from build123d import *

# Parameters (mm, degrees)
SKETCH1_R                 = 36
BIG_END_DEPTH             = 11
SKETCH2_R                 = 18
SMALL_END_DEPTH           = 11
BEAM_DEPTH                = 11
CAP_BOLT_BOSSES_DEPTH     = 11
BEAM_START                = 7
BEAM_POCKET_FRONT_DEPTH   = 5
BEAM_START_2              = -12
BEAM_POCKET_REAR_DEPTH    = 5
BIG_END_BORE_DEPTH        = 178.709988464
BIG_END_BORE_DEPTH_BACK   = 178.709988464
SKETCH7_R                 = 26.75
SMALL_END_BORE_DEPTH      = 178.709988464
SMALL_END_BORE_DEPTH_BACK = 178.709988464
SKETCH8_R                 = 11.85


with BuildPart() as part:
    # Sketch1 → Big End (new, symmetric)
    with BuildSketch(Plane.XY):
        Circle(SKETCH1_R)
    extrude(amount=BIG_END_DEPTH, both=True)



with BuildPart() as body_2:
    # Sketch2 → Small End (new, symmetric)
    with BuildSketch(Plane.XY):
        with Locations((0, 154.8)):
            Circle(SKETCH2_R)
    extrude(amount=SMALL_END_DEPTH, both=True)


with BuildPart() as part_1:
    add(part.part)

    add(body_2.part)  # Beam merges body 2
    # Sketch3 → Beam (add, symmetric)
    with BuildSketch(Plane.XY):
        Polygon((-15, 20), (15, 20), (10, 142.8), (-10, 142.8), align=None)
    extrude(amount=BEAM_DEPTH, both=True)

    # Sketch4 → Cap Bolt Bosses (add, symmetric)
    with BuildSketch(Plane.XY):
        with BuildLine():
            Line((29, -9), (37, -9))
            ThreePointArc((37, -9), (39.121320344, -8.121320344), (40, -6))
            Line((40, -6), (40, 9))
            ThreePointArc((40, 9), (39.121320344, 11.121320344), (37, 12))
            Line((37, 12), (29, 12))
            ThreePointArc((29, 12), (26.878679656, 11.121320344), (26, 9))
            Line((26, 9), (26, -6))
            ThreePointArc((26, -6), (26.878679656, -8.121320344), (29, -9))
        make_face()
        with BuildLine():
            Line((-37, -9), (-29, -9))
            ThreePointArc((-29, -9), (-26.878679656, -8.121320344), (-26, -6))
            Line((-26, -6), (-26, 9))
            ThreePointArc((-26, 9), (-26.878679656, 11.121320344), (-29, 12))
            Line((-29, 12), (-37, 12))
            ThreePointArc((-37, 12), (-39.121320344, 11.121320344), (-40, 9))
            Line((-40, 9), (-40, -6))
            ThreePointArc((-40, -6), (-39.121320344, -8.121320344), (-37, -9))
        make_face()
    extrude(amount=CAP_BOLT_BOSSES_DEPTH, both=True)

    # Sketch5 → Beam Pocket Front (cut)
    with BuildSketch(Plane.XY.offset(BEAM_START)):
        with BuildLine():
            Line((-5.386546762, 44), (5.386546762, 44))
            ThreePointArc((5.386546762, 44), (7.546862517, 44.918405458), (8.384481085, 47.111309443))
            Line((8.384481085, 47.111309443), (5.607253362, 121.911309443))
            ThreePointArc((5.607253362, 121.911309443), (4.69091358, 123.960315756), (2.609319039, 124.8))
            Line((2.609319039, 124.8), (-2.609319039, 124.8))
            ThreePointArc((-2.609319039, 124.8), (-4.69091358, 123.960315756), (-5.607253362, 121.911309443))
            Line((-5.607253362, 121.911309443), (-8.384481085, 47.111309443))
            ThreePointArc((-8.384481085, 47.111309443), (-7.546862517, 44.918405458), (-5.386546762, 44))
        make_face()
    extrude(amount=BEAM_POCKET_FRONT_DEPTH, mode=Mode.SUBTRACT)

    # Sketch6 → Beam Pocket Rear (cut)
    with BuildSketch(Plane.XY.offset(BEAM_START_2)):
        with BuildLine():
            Line((-5.386546762, 44), (5.386546762, 44))
            ThreePointArc((5.386546762, 44), (7.546862517, 44.918405458), (8.384481085, 47.111309443))
            Line((8.384481085, 47.111309443), (5.607253362, 121.911309443))
            ThreePointArc((5.607253362, 121.911309443), (4.69091358, 123.960315756), (2.609319039, 124.8))
            Line((2.609319039, 124.8), (-2.609319039, 124.8))
            ThreePointArc((-2.609319039, 124.8), (-4.69091358, 123.960315756), (-5.607253362, 121.911309443))
            Line((-5.607253362, 121.911309443), (-8.384481085, 47.111309443))
            ThreePointArc((-8.384481085, 47.111309443), (-7.546862517, 44.918405458), (-5.386546762, 44))
        make_face()
    extrude(amount=BEAM_POCKET_REAR_DEPTH, mode=Mode.SUBTRACT)

    # Sketch7 → Big End Bore (cut, two sides: drawn at the far end of the back side and taken through both)
    with BuildSketch(Plane.XY.offset(-BIG_END_BORE_DEPTH_BACK)):
        Circle(SKETCH7_R)
    extrude(amount=BIG_END_BORE_DEPTH + BIG_END_BORE_DEPTH_BACK, mode=Mode.SUBTRACT)

    # Sketch8 → Small End Bore (cut, two sides: drawn at the far end of the back side and taken through both)
    with BuildSketch(Plane.XY.offset(-SMALL_END_BORE_DEPTH_BACK)):
        with Locations((0, 154.8)):
            Circle(SKETCH8_R)
    extrude(amount=SMALL_END_BORE_DEPTH + SMALL_END_BORE_DEPTH_BACK, mode=Mode.SUBTRACT)


solid = part_1.part
Work out the finished part from the listing and answer in its coordinate system (mm). A direction names the side the tool comes from. Give positions to 0.01 mm unless a question says otherwise; leave off trailing zeros. Loops run counter-clockwise (first coordinate to the right, second up) from the corner with the lowest first, then second, coordinate; pieces in that order, holes last. Notation, with made-up numbers: (83.25, -28.5) -> (105.25, -28.5) arc R24 cw to (105.25, -14.5) -> close; hole circle Ø4 at (-23, 16.25). An arc over 180 degrees is marked (long way). Use a Markdown table: item, result. Add a question column.
1) Consider line 1 along Y through (x, z) = (0, 2.5); line 2 along X through (y, z) = (0, 4); line 3 along X through (y, z) = (154.8, -1.75). Determine where each line is inside the solid, lowest interval first.
2) The part is cut by section C-C, the plane x = -20. Determine the outline of the cut face in (y, z).
3) Which of the six approach directions +Z, -Z, +X, -X, +Y, -Y give full straight-line access (tool end or side, diameter ignored) to faces 4 (the flat face through (0, 85, -7)), 5 (the flat face through (-12.264, 87.186, 0.154)), 6 (the flat face through (0, 44, 9))?
4) The part is cut by section B-B, the plane z = 0. Determine the outline of the cut face in (x, y), plus the area to 3 significant figures.
5) The part is cut by section A-A, the plane y = 154.8. Determine the outline of the cut face in (x, z).
6) Each of these flat-tipped pins is pushed along its axis until it touches: P1, Ø1, axis at x = -19, z = -6, coming from the -Y side; P2, Ø1.5, axis at y = 125, z = -0.5, coming from the +X side; P3, Ø2, axis at x = 4, y = 146.5, coming from the +Z side; P4, Ø8.5, axis at x = 2.5, y = 68.5, coming from the -Z side. Where does it stop, or does it pass through?
7) For a pull along X with two mould halves and no side action, classify faces 1 (the flat face through (12.325, 85.689, 0.154)), 2 (the flat face through (0, 44, -9)), 3 (the flat face through (-9, 53, 11)) as +X half, -X half, draft (parallel to the pull), parting line (faces both ways), or undercut.
Reported:
| question | item | result |
|---|---|---|
| 1 | line 1 | y = -36 to -26.75, 26.75 to 142.95, 166.65 to 172.8 |
| 1 | line 2 | x = -40 to -26.75, 26.75 to 40 |
| 1 | line 3 | x = -18 to -11.85, 11.85 to 18 |
| 2 | outline | (-29.93, -11) -> (-17.76, -11) -> (-17.76, 11) -> (-29.93, 11) -> close; (17.76, -11) -> (29.93, -11) -> (29.93, 11) -> (17.76, 11) -> close |
| 3 | face 4 | -Z |
| 3 | face 5 | +Z, -Z, -X |
| 3 | face 6 | +Z |
| 4 | outline | (-40, -6) arc R3 ccw to (-37, -9) -> (-34.86, -9) arc R36 ccw to (34.86, -9) -> (37, -9) arc R3 ccw to (40, -6) -> (40, 9) arc R3 ccw to (37, 12) -> (33.94, 12) arc R36 ccw to (14.47, 32.96) -> (10.12, 139.91) arc R18 ccw (long way) to (-10.12, 139.91) -> (-14.47, 32.96) arc R36 ccw to (-33.94, 12) -> (-37, 12) arc R3 ccw to (-40, 9) -> close; hole circle Ø53.5 at (0, 0); hole circle Ø23.7 at (0, 154.8) |
| 4 | area | 5,110 mm^2 |
| 5 | outline | (-18, -11) -> (-11.85, -11) -> (-11.85, 11) -> (-18, 11) -> close; (11.85, -11) -> (18, -11) -> (18, 11) -> (11.85, 11) -> close |
| 6 | P1 | stops at y = -30.88 |
| 6 | P2 | stops at x = 10.76 |
| 6 | P3 | passes through |
| 6 | P4 | stops at z = -7 |
| 7 | face 1 | +X half |
| 7 | face 2 | undercut |
| 7 | face 3 | draft |
